```python
from build123d import *


with BuildPart() as f1:
    # F0 (on Front) → F1 (revolve)
    with BuildSketch(Plane.XZ):
        with BuildLine():
            Line((-12.820962, 242.57), (-7.355597, 237.104635))
            Line((-7.355597, 237.104635), (0, 239.075561))
            Line((0, 239.075561), (0, 240.829671))
            Line((0, 240.829671), (0, 245.209498))
            Line((0, 245.209498), (0, 246.18163))
            Line((0, 246.18163), (0, 247.46631))
            ThreePointArc((0, 247.46631), (-3.923627, 249.786079), (-7.92797, 251.963556))
            ThreePointArc((-7.92797, 251.963556), (-8.440309, 252.156449), (-8.983817, 252.222))
            Line((-8.983817, 252.222), (-16.967452, 252.222))
            ThreePointArc((-16.967452, 252.222), (-17.423207, 252.267892), (-17.860664, 252.403726))
            Line((-17.860664, 252.403726), (-29.76303, 257.45598))
            Line((-29.76303, 257.45598), (-31.251715, 253.948857))
            Line((-31.251715, 253.948857), (-41.773086, 258.414914))
            Line((-41.773086, 258.414914), (-40.2844, 261.922037))
            Line((-40.2844, 261.922037), (-43.2816, 263.194273))
            ThreePointArc((-43.2816, 263.194273), (-47.440371, 265.06445), (-51.6636, 266.784125))
            Line((-51.6636, 266.784125), (-52.299364, 266.148361))
            ThreePointArc((-52.299364, 266.148361), (-52.391699, 266.086665), (-52.500615, 266.065))
            Line((-52.500615, 266.065), (-54.325387, 266.065))
            ThreePointArc((-54.325387, 266.065), (-54.526639, 266.148361), (-54.61, 266.349613))
            Line((-54.61, 266.349613), (-54.61, 284.802049))
            Line((-54.61, 284.802049), (-74.180059, 285.188049))
            Line((-74.180059, 285.188049), (-74.180059, 250.422508))
            Line((-74.180059, 250.422508), (-61.449014, 250.422508))
            Line((-61.449014, 250.422508), (-50.676592, 255.319059))
            Line((-50.676592, 255.319059), (-24.13, 242.57))
            Line((-24.13, 242.57), (-13.944356, 242.57))
            Line((-13.944356, 242.57), (-12.820962, 242.57))
        make_face()
    revolve(axis=Axis((15.058352, 0, 0), (1, 0, 0)))


solid = f1.part
```
Part model, mm, in its own coordinate system. A direction names the side the tool comes from. Round coordinates to 2 decimals unless told otherwise and drop trailing zeros.
Item 1: Two-plate mould, pull along Z, no slides. Class faces 1 (the conical face through (-18.61, -75.91, 241.05)), 2 (the flat face through (0, -203, 129)), 3 (the cylindrical face through (-67.73, 222.17, 115.55)): +Z half, -Z half, draft (parallel to the pull), parting line (faces both ways), or undercut.
Results:
face 1: parting line
face 2: draft
face 3: undercut
Item 2: Which spindle directions (+Z, -Z, +X, -X, +Y, -Y) get a long thin tool onto all of the face, cutting with end or side? Do faces 4 (the flat face through (-74.18, 252, -1)), 5 (the conical face through (-31.18, -251.96, -33.08)), 6 (the cylindrical face through (-13.032, 153.473, -200.155)), 7 (the cylindrical face through (-18.4, -72.86, 231.37)). Say none if no direction does.
Results:
face 4: +Z, -Z, -X, +Y, -Y
face 5: none
face 6: +X
face 7: -X
Item 3: Probe L1, parallel to Y at x = -17, z = 0; L2, parallel to Z at x = -40.5, y = -36; L3, parallel to Z at x = -70, y = 0. List the from-to ranges inside material, lowest first.
Results:
L1: y = -252.22 to -242.57, 242.57 to 252.22
L2: z = -259.53 to -258.92, -255.35 to -247.83, 247.83 to 255.35, 258.92 to 259.53
L3: z = -285.11 to -250.42, 250.42 to 285.11
Item 4: Drop flat-ended pins along their axis: pin 1 Ø8 at (x, z) = (-56.5, 150) entering from +Y; pin 2 Ø6 at (x, z) = (-8, -78) entering from -Y; pin 3 Ø4 at (x, z) = (-48, 156.5) entering from -Y. Give the stop position or say it passes through.
Results:
pin 1: stops at y = 244.58
pin 2: stops at y = -240.77
pin 3: stops at y = -216
